Could you check a few things on this drawing? It's one solid part, dimensions in mm from its lowest x, y, z. A direction names the side the tool comes from. Give positions to 0.01 mm unless a question says otherwise; leave off trailing zeros. Order: outer loops, then holes, each group sorted by start corner. A loop starts at its lowest first (then second) coordinate and runs counter-clockwise, first axis right, second up. Notation, with made-up numbers: M 8,-24.75 L 20,-24.75 A18 ccw 20,-2.75 Z; hole C 24,-35 d1. An arc over 180 degrees is marked long. Use one line per item in the form item = value. Start each with the question number.
1. I want a section at C-C, the plane y = 23. List the corners of the cut face in (x, z) for me.
2. I want a section at A-A, the plane z = 5. List the corners of the cut face in (x, y) for me, and give its area (3 significant figures).
3. For the marked faces 1, 2 and 3, which set-ups out of +Z, -Z, +X, -X, +Y, -Y let a thin tool reach every point of the face, with its end or its side?
4. I want a section at B-B, the plane x = 32.5. List the corners of the cut face in (y, z) for me.
5. I want a section at D-D, the plane z = 8. List the corners of the cut face in (x, y) for me.
6. We'd pull the mould along Z, two halves only. Please class the marked faces 4, 5, 6 and 7: +Z half, -Z half, draft (parallel to the pull), parting line (faces both ways), or undercut.
7. I need wall thicknesses on L1, parallel to Y at x = 27, z = 5; L2, parallel to X at y = 30.5, z = 11.75; L3, parallel to X at y = 19, z = 6. Which ranges of each line are inside material? Lowest first, please.
8. Will these pins go through, and if not, where does the flat tip stop? P1, Ø0.5, axis at x = 0.5, z = 7.5, coming from the -Y side; P2, Ø0.8, axis at x = 0.5, y = 32, coming from the -Z side; P3, Ø3, axis at x = 9, z = 6.5, coming from the +Y side.
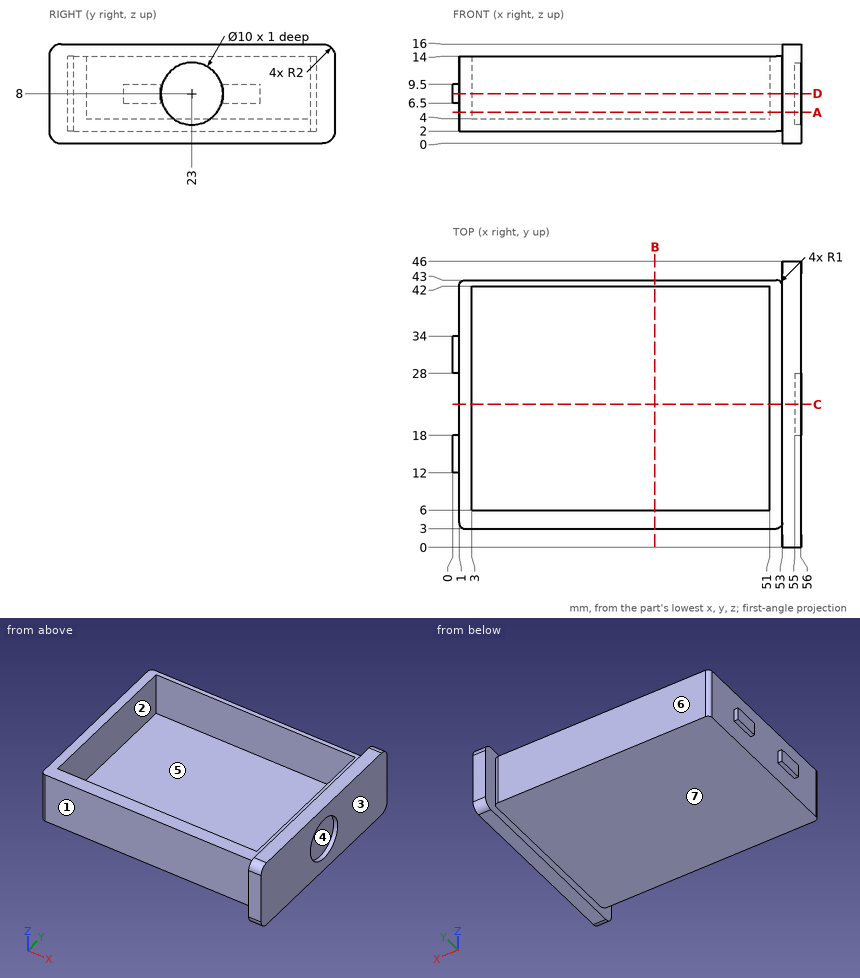
Check result:
q1.outline = M 1,2 L 53,2 L 53,0 L 56,0 L 56,3 L 55,3 L 55,13 L 56,13 L 56,16 L 53,16 L 53,14 L 51,14 L 51,4 L 3,4 L 3,14 L 1,14 Z
q2.outline = M 1,4 A1 ccw 2,3 L 52,3 A1 ccw 53,4 L 53,0 L 56,0 L 56,19 L 55,19 L 55,27 L 56,27 L 56,46 L 53,46 L 53,42 A1 ccw 52,43 L 2,43 A1 ccw 1,42 Z; hole M 3,6 L 51,6 L 51,42 L 3,42 Z
q2.area = 481 mm2
q3.face_1 = +Z, -Z, -X, -Y
q3.face_2 = +Z
q3.face_3 = +Z, -Z, +X, +Y, -Y
q4.outline = M 3,2 L 43,2 L 43,14 L 42,14 L 42,4 L 6,4 L 6,14 L 3,14 Z
q5.outline = M 0,12 L 1,12 L 1,4 A1 ccw 2,3 L 52,3 A1 ccw 53,4 L 53,0 L 56,0 L 56,18 L 55,18 L 55,28 L 56,28 L 56,46 L 53,46 L 53,42 A1 ccw 52,43 L 2,43 A1 ccw 1,42 L 1,34 L 0,34 L 0,28 L 1,28 L 1,18 L 0,18 Z; hole M 3,6 L 51,6 L 51,42 L 3,42 Z
q6.face_4 = undercut
q6.face_5 = +Z half
q6.face_6 = draft
q6.face_7 = -Z half
q7.L1 = 3 to 6, 42 to 43
q7.L2 = 1 to 3, 51 to 56
q7.L3 = 1 to 3, 51 to 55
q8.P1 = 12
q8.P2 = 6.5
q8.P3 = 43
